```python
from build123d import *

# Parameters (mm, degrees)
SKETCH_1_R          = 19.75
SKETCH_1_R_2        = 18.75
EXTRUDE_1_DEPTH     = 1
SKETCH_2_R          = 19.75
EXTRUDE_2_DEPTH     = 41.8
SKETCH_3_R          = 10
SKETCH_3_R_2        = 1.25
CUT_EXTRUDE_1_DEPTH = 13
SKETCH_4_R          = 2
EXTRUDE_3_DEPTH     = 1
SKETCH_5_R          = 2
EXTRUDE_4_DEPTH     = 1
SKETCH_6_R          = 3
CUT_EXTRUDE_2_DEPTH = 6
EXTRUDE_START       = -42.8
EXTRUDE_5_DEPTH     = 42.8
SKETCH_9_R          = 25
CUT_EXTRUDE_4_DEPTH = 0.25


with BuildPart() as part:
    # 草图1 → 凸台-拉伸1 (new body)
    with BuildSketch(Plane(origin=(0, 0, 0), x_dir=(1, 0, 0), z_dir=(0, 1, 0))):
        with Locations(Location((0, 0, 0), (0, 0, 270))):
            Circle(SKETCH_1_R)
        with Locations(Location((0, 0, 0), (0, 0, 270))):
            Circle(SKETCH_1_R_2, mode=Mode.SUBTRACT)
    extrude(amount=EXTRUDE_1_DEPTH)

    # 草图2 → 凸台-拉伸2 (add)
    with BuildSketch(Plane(origin=(0, 1, 0), x_dir=(1, 0, 0), z_dir=(0, 1, 0))):
        with Locations(Location((0, 0, 0), (0, 0, 270))):
            Circle(SKETCH_2_R)
    extrude(amount=EXTRUDE_2_DEPTH)

    # 草图3 → 切除-拉伸1 (cut)
    with BuildSketch(Plane(origin=(0, 42.8, 0), x_dir=(1, 0, 0), z_dir=(0, 1, 0))):
        with Locations(Location((0, 0, 0), (0, 0, 270))):
            Circle(SKETCH_3_R)
        with Locations(Location((0, 13.5, 0), (0, 0, 270))):
            Circle(SKETCH_3_R_2)
        with Locations(Location((11.691342951, 6.75, 0), (0, 0, 270))):
            Circle(SKETCH_3_R_2)
        with Locations(Location((11.691342951, -6.75, 0), (0, 0, 270))):
            Circle(SKETCH_3_R_2)
        with Locations(Location((0, -13.5, 0), (0, 0, 270))):
            Circle(SKETCH_3_R_2)
        with Locations(Location((-11.691342951, -6.75, 0), (0, 0, 270))):
            Circle(SKETCH_3_R_2)
        with Locations(Location((-11.691342951, 6.75, 0), (0, 0, 270))):
            Circle(SKETCH_3_R_2)
    extrude(amount=-CUT_EXTRUDE_1_DEPTH, mode=Mode.SUBTRACT)

    # 草图4 → 凸台-拉伸3 (add)
    with BuildSketch(Plane.XZ.offset(-1)):
        with Locations(Location((12, 0, 0), (0, 0, 90))):
            Circle(SKETCH_4_R)
        with Locations(Location((-6, -10.392304845, 0), (0, 0, 90))):
            Circle(SKETCH_4_R)
        with Locations(Location((-6, 10.392304845, 0), (0, 0, 90))):
            Circle(SKETCH_4_R)
    extrude(amount=EXTRUDE_3_DEPTH)

    # 草图5 → 凸台-拉伸4 (add)
    with BuildSketch(Plane(origin=(0, 42.8, 0), x_dir=(1, 0, 0), z_dir=(0, 1, 0))):
        with Locations(Location((13.5, 0, 0), (0, 0, 270))):
            Circle(SKETCH_5_R)
        with Locations(Location((6.75, -11.691342951, 0), (0, 0, 270))):
            Circle(SKETCH_5_R)
        with Locations(Location((-6.75, -11.691342951, 0), (0, 0, 270))):
            Circle(SKETCH_5_R)
        with Locations(Location((-13.5, 0, 0), (0, 0, 270))):
            Circle(SKETCH_5_R)
        with Locations(Location((-6.75, 11.691342951, 0), (0, 0, 270))):
            Circle(SKETCH_5_R)
        with Locations(Location((6.75, 11.691342951, 0), (0, 0, 270))):
            Circle(SKETCH_5_R)
    extrude(amount=EXTRUDE_4_DEPTH)

    # 草图6 → 切除-拉伸2 (cut)
    with BuildSketch(Plane.XZ.offset(-1)):
        with Locations(Location((-13.5, 0, 0), (0, 0, 270))):
            Circle(SKETCH_6_R)
        with Locations(Location((6.75, 11.691342951, 0), (0, 0, 270))):
            Circle(SKETCH_6_R)
        with Locations(Location((6.75, -11.691342951, 0), (0, 0, 270))):
            Circle(SKETCH_6_R)
    extrude(amount=-CUT_EXTRUDE_2_DEPTH, mode=Mode.SUBTRACT)

    # 草图7 → 凸台-拉伸5 (add)
    with BuildSketch(Plane(origin=(0, 42.8, 0), x_dir=(1, 0, 0), z_dir=(0, 1, 0)).offset(EXTRUDE_START)):
        with BuildLine():
            ThreePointArc((21.75, 0), (21.563925735, 2.838944681), (21.008886722, 5.629314231))
            Line((21.008886722, 5.629314231), (19.077035069, 5.111676141))
            ThreePointArc((19.077035069, 5.111676141), (19.581036012, 2.577892296), (19.75, 0))
            ThreePointArc((19.75, 0), (15.668728471, -12.023038223), (5.111676141, -19.077035069))
            Line((5.111676141, -19.077035069), (5.629314231, -21.008886722))
            ThreePointArc((5.629314231, -21.008886722), (17.255435151, -13.240561081), (21.75, 0))
        make_face()
    extrude(amount=EXTRUDE_5_DEPTH)

    # 草图9 → 切除-拉伸4 (cut)
    with BuildSketch(Plane.XZ):
        Circle(SKETCH_9_R)
    extrude(amount=-CUT_EXTRUDE_4_DEPTH, mode=Mode.SUBTRACT)


solid = part.part
```
The model under review builds one solid part; all positions refer to its coordinate system, in mm. A direction names the side the tool comes from. Round coordinates to 2 decimals unless told otherwise and drop trailing zeros. Loops run counter-clockwise (first coordinate to the right, second up) from the corner with the lowest first, then second, coordinate; pieces in that order, holes last. Notation, with made-up numbers: M -32,8.25 L 22,8.25 A16 ccw 22,28.25 Z; hole C 50,40.5 d11. An arc over 180 degrees is marked long. Write item = value, one per line.
Item 1: Take a section at D-D on z = -6.75. Write out the cut boundary in (x, y), then the cut area to 3 significant figures.
Return value:
outline = M -18.56,0.25 L -17.49,0.25 L -17.49,1 L 17.49,1 L 17.49,0.25 L 18.56,0.25 L 18.56,42.8 L 12.94,42.8 L 12.94,29.8 L 10.44,29.8 L 10.44,42.8 L 7.38,42.8 L 7.38,29.8 L -7.38,29.8 L -7.38,42.8 L -10.44,42.8 L -10.44,29.8 L -12.94,29.8 L -12.94,42.8 L -18.56,42.8 Z
area = 1,300 mm2
Item 2: Take a section at C-C on y = 20. Write out the cut boundary in (x, z).
Return value:
outline = M 5.11,19.08 A19.75 ccw long 19.08,-5.11 L 21.01,-5.63 A21.75 ccw 5.63,21.01 Z
Item 3: Machinability: for faces 1 (the cylindrical face through (4.925, 3.958, -9.311)), 2 (the flat face through (14, 43.8, 0)), 3 (the flat face through (0, 29.8, 13)), which of the approach directions +Z, -Z, +X, -X, +Y, -Y give a long, thin tool a straight path to every point of the face, cutting with its end or side? Answer none if there is none.
Return value:
face_1 = -Y
face_2 = +Z, -Z, +X, -X, +Y
face_3 = +Y
Item 4: Take a section at B-B on x = 6.75. Write out the cut boundary in (y, z), then the cut area to 3 significant figures.
Return value:
outline = M 0.25,-18.56 L 42.8,-18.56 L 42.8,-13.69 L 43.8,-13.69 L 43.8,-9.69 L 42.8,-9.69 L 42.8,-7.38 L 29.8,-7.38 L 29.8,7.38 L 42.8,7.38 L 42.8,9.69 L 43.8,9.69 L 43.8,13.69 L 42.8,13.69 L 42.8,20.68 L 0.25,20.68 L 0.25,17.49 L 1,17.49 L 1,14.69 L 7,14.69 L 7,8.69 L 1,8.69 L 1,-8.69 L 7,-8.69 L 7,-14.69 L 1,-14.69 L 1,-17.49 L 0.25,-17.49 Z
area = 1,390 mm2
Item 5: Insertion check: P1, Ø3, axis at x = 9.5, y = 39, coming from the +Z side; P2, Ø5, axis at y = 31.5, z = 11, coming from the +X side; P3, Ø5, axis at x = 7.5, z = 11.5, coming from the -Y side. Each pin has a flat end and moves straight along its axis. Give the tip position at first contact, or say it passes through.
Return value:
P1 = 20.23
P2 = 20.02
P3 = 1
Item 6: For line 1 (Y direction, x = -11, z = 0); line 2 (Y direction, x = -2.5, z = -2); line 3 (X direction, y = 33, z = -6.5), list the stretches that pass through material, from the lowest coordinate up. Write a range as [from, to].
Return value:
line_1 = [7, 42.8]
line_2 = [1, 29.8]
line_3 = [-18.65, -12.92], [-10.47, -7.6], [7.6, 10.47], [12.92, 18.65]
Item 7: Take a section at A-A on y = 39.5. Write out the cut boundary in (x, z).
Return value:
outline = M 5.11,19.08 A19.75 ccw long 19.08,-5.11 L 21.01,-5.63 A21.75 ccw 5.63,21.01 Z; hole C -11.69,-6.75 d2.5; hole C -11.69,6.75 d2.5; hole C 0,0 d20; hole C 0,-13.5 d2.5; hole C 0,13.5 d2.5; hole C 11.69,-6.75 d2.5; hole C 11.69,6.75 d2.5
